Read the model definition and answer for the solid it produces. Units are mm, in the model's axes. A direction names the side the tool comes from. Coordinates: 2 decimals unless noted, no trailing zeros. Write each loop counter-clockwise with the first axis right and the second up, starting at its lowest first coordinate (ties: lowest second). Pieces come first, ordered by that corner, then holes. Notation, with made-up numbers: (51, -24.75) -> (109, -24.75) arc R15 ccw to (109, -1.75) -> close; hole circle Ø9 at (5.5, -12). An arc over 180 degrees is marked (long way). One line per item, written item: value. Start each with the question number.
from build123d import *

# Parameters (mm, degrees)
SKETCH_1_W          = 60
SKETCH_1_H          = 55
SKETCH_1_R          = 11
SKETCH_1_R_2        = 1.5
EXTRUDE_1_DEPTH     = 5
EXTRUDE_2_DEPTH     = 35
SKETCH_4_R          = 3
CUT_EXTRUDE_1_DEPTH = 5
CUT_EXTRUDE_2_REACH = 92.692


with BuildPart() as part:
    # Эскиз1 → Бобышка-Вытянуть1 (new body)
    with BuildSketch(Plane(origin=(0, 0, 0), x_dir=(1, 0, 0), z_dir=(0, 1, 0))):
        with Locations((30, 27.5)):
            Rectangle(SKETCH_1_W, SKETCH_1_H)
        with Locations(Location((30, 21.5, 0), (0, 0, 270))):
            Circle(SKETCH_1_R, mode=Mode.SUBTRACT)
        with Locations(Location((14.5, 37, 0), (0, 0, 270))):
            Circle(SKETCH_1_R_2, mode=Mode.SUBTRACT)
        with Locations(Location((45.5, 37, 0), (0, 0, 270))):
            Circle(SKETCH_1_R_2, mode=Mode.SUBTRACT)
        with Locations(Location((45.5, 6, 0), (0, 0, 270))):
            Circle(SKETCH_1_R_2, mode=Mode.SUBTRACT)
        with Locations(Location((14.5, 6, 0), (0, 0, 270))):
            Circle(SKETCH_1_R_2, mode=Mode.SUBTRACT)
    extrude(amount=EXTRUDE_1_DEPTH)

    # Эскиз3 → Бобышка-Вытянуть2 (add)
    with BuildSketch(Plane(origin=(0, 5, 0), x_dir=(1, 0, 0), z_dir=(0, 1, 0))):
        Polygon((5, 50), (55, 50), (55, 0), (60, 0), (60, 55), (0, 55), (0, 0), (5, 0), align=None)
    extrude(amount=EXTRUDE_2_DEPTH)

    # Эскиз4 → Вырез-Вытянуть1 (cut)
    with BuildSketch(Plane(origin=(0, 0, -55), x_dir=(-1, 0, 0), z_dir=(0, 0, -1))):
        with Locations((-12.5, 10)):
            Circle(SKETCH_4_R)
        with Locations((-12.5, 30)):
            Circle(SKETCH_4_R)
        with Locations((-47.5, 30)):
            Circle(SKETCH_4_R)
        with Locations((-47.5, 10)):
            Circle(SKETCH_4_R)
    extrude(amount=-CUT_EXTRUDE_1_DEPTH, mode=Mode.SUBTRACT)

    # Вырез-Вытянуть2: up to this face of the body (flat: up to its plane)
    cut_extrude_2_end = Plane(part.part.faces().sort_by_distance((60, 20, -27.5))[0])
    # Эскиз5 → Вырез-Вытянуть2 (cut, up to the picked face)
    with BuildSketch(Plane.ZY, mode=Mode.PRIVATE) as cut_extrude_2_sk1:
        Polygon((0, 5), (-50, 40), (0, 40), align=None)
    cut_extrude_2_tool1 = split(extrude(cut_extrude_2_sk1.sketch, amount=-CUT_EXTRUDE_2_REACH, mode=Mode.PRIVATE), bisect_by=cut_extrude_2_end, keep=Keep.BOTH, mode=Mode.PRIVATE)
    add(cut_extrude_2_tool1.solids().sort_by(Axis((0, 28.333333, -16.666667), (1, 0, 0)))[0], mode=Mode.SUBTRACT)


solid = part.part
1. Find the intervals of material crossed by probe 1 along Y at (x, z) = (47.5, -51.2); probe 2 along X at (y, z) = (3.3, -21.5); probe 3 along Z at (x, y) = (45, 2), in increasing order. Write a range as from..to.
2. A tool of negligible diameter and unlimited length cuts with its end or side. For faces 5 (the face through (2.465, 22.255, -24.65)), 6 (the face through (55, 18, -31)), from which of +Z, -Z, +X, -X, +Y, -Y can it reach the whole face along a straight path? Write none if from no direction.
3. A cutting plane is placed at B-B on x = 39. Give the vertices of the cut face in (y, z).
4. Given pin 1 (4 mm diameter, centred on x = 41, y = 17.5, fed in from +Z); pin 2 (10.5 mm diameter, centred on y = 14.5, z = -36.5, fed in from -X); pin 3 (6 mm diameter, centred on x = 25, z = -14.5, fed in from +Y), each flat-ended and moving along its own axis, determine where each tip first touches the part or whether it passes through.
5. A cutting plane is placed at D-D on z = -21. Give the vertices of the cut face in (x, y), then the cut area to 3 significant figures.
6. For a pull along Y with two mould halves and no side action, classify faces 1 (the face through (30, 0, -34)), 2 (the face through (50.5, 30.1, -52.5)), 3 (the face through (13.6, 2.5, -38.2)), 4 (the face through (14.71, 32.03, -52.54)) as +Y half, -Y half, draft (parallel to the pull), parting line (faces both ways), or undercut.
7. A cutting plane is placed at C-C on y = 12. Give the vertices of the cut face in (x, z).
8. A cutting plane is placed at A-A on z = -37. Give the vertices of the cut face in (x, y).
Derived:
1. probe 1: y = 0..7, 13..27, 33..40
1. probe 2: x = 0..19, 41..60
1. probe 3: z = -55..-38.41, -35.59..-7.41, -4.59..0
2. face 5: +Z, +X, -X, +Y
2. face 6: +Z, +Y
3. outline: (0, -55) -> (40, -55) -> (40, -50) -> (5, -50) -> (5, -27.82) -> (0, -27.82) -> close; (0, -15.18) -> (5, -15.18) -> (5, 0) -> (0, 0) -> close
4. pin 1: stops at z = -50
4. pin 2: stops at x = 0
4. pin 3: stops at y = 5
5. outline: (0, 0) -> (19.01, 0) -> (19.01, 5) -> (5, 5) -> (5, 19.7) -> (0, 19.7) -> close; (40.99, 0) -> (60, 0) -> (60, 19.7) -> (55, 19.7) -> (55, 5) -> (40.99, 5) -> close
5. area: 337 mm2
6. face 1: -Y half
6. face 2: undercut
6. face 3: draft
6. face 4: undercut
7. outline: (0, -55) -> (10.26, -55) -> (10.26, -50) -> (5, -50) -> (5, -10) -> (0, -10) -> close; (14.74, -55) -> (45.26, -55) -> (45.26, -50) -> (14.74, -50) -> close; (49.74, -55) -> (60, -55) -> (60, -10) -> (55, -10) -> (55, -50) -> (49.74, -50) -> close
8. outline: (0, 0) -> (13, 0) -> (13, 5) -> (5, 5) -> (5, 30.9) -> (0, 30.9) -> close; (16, 0) -> (44, 0) -> (44, 5) -> (16, 5) -> close; (47, 0) -> (60, 0) -> (60, 30.9) -> (55, 30.9) -> (55, 5) -> (47, 5) -> close
